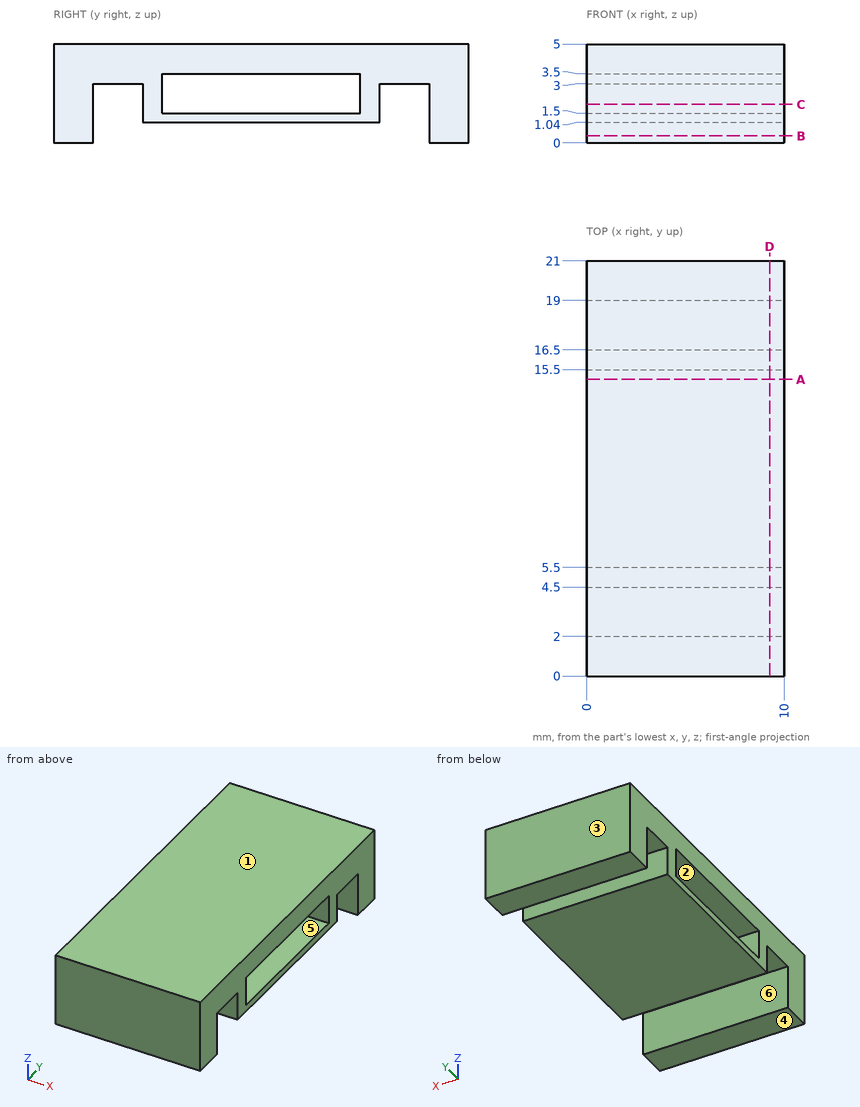
Part print with two shaded views. Sizes in mm from the minimum x, y, z corner. A direction names the side the tool comes from. Round coordinates to 2 decimals unless told otherwise and drop trailing zeros. Order: outer loops, then holes, each group sorted by start corner. A loop starts at its lowest first (then second) coordinate and runs counter-clockwise, first axis right, second up.
(1) Drill centre lines: line 1 (Y direction, x = 8, z = 2.7); line 2 (Y direction, x = 4.25, z = 1.2); line 3 (Z direction, x = 5, y = 10). Where is each one in solid material? Low to high.
(2) Pin check, flat tips, straight feed: pin 1 (0.8 mm diameter, centred on x = 4, y = 3, fed in from -Z); pin 2 (2 mm diameter, centred on x = 3.5, y = 4, fed in from -Z). Stop position of each tip, or through.
(3) Pull direction Z, two halves, no side cores. Call the marked faces 1, 2 and 3: released by +Z, released by -Z, zero draft, split by the parting line, or undercut.
(4) Band-saw the part on B-B (z = 0.35). List the corners of the cut face in (x, y), then the cut area to 3 significant figures.
(5) 3-axis set-ups, long thin cutter, end or side, ignore diameter. For the marked faces 4, 5 and 6: which of +Z, -Z, +X, -X, +Y, -Y reach the whole face in a straight line?
(6) Band-saw the part on D-D (x = 9.25). List the corners of the cut face in (y, z), then the cut area to 3 significant figures.
(7) Band-saw the part on C-C (z = 1.95). List the corners of the cut face in (x, y).
(8) Band-saw the part on A-A (y = 15). List the corners of the cut face in (x, z), then the cut area to 3 significant figures.
Verdict:
1. line 1: y = 0 to 2, 4.5 to 5.5, 15.5 to 16.5, 19 to 21
1. line 2: y = 0 to 2, 4.5 to 16.5, 19 to 21
1. line 3: z = 1.04 to 1.5, 3.5 to 5
2. pin 1: stops at z = 3
2. pin 2: stops at z = 1.04
3. face 1: released by +Z
3. face 2: undercut
3. face 3: zero draft
4. outline: (0, 0) - (10, 0) - (10, 2) - (0, 2) - close; (0, 19) - (10, 19) - (10, 21) - (0, 21) - close
4. area: 40.0 mm2
5. face 4: -Z, +X, -X, +Y, -Y
5. face 5: +X, -X
5. face 6: -Z, +X, -X
6. outline: (0, 0) - (2, 0) - (2, 3) - (4.5, 3) - (4.5, 1.04) - (16.5, 1.04) - (16.5, 3) - (19, 3) - (19, 0) - (21, 0) - (21, 5) - (0, 5) - close; hole (5.5, 1.5) - (15.5, 1.5) - (15.5, 3.5) - (5.5, 3.5) - close
6. area: 57.5 mm2
7. outline: (0, 0) - (10, 0) - (10, 2) - (0, 2) - close; (0, 4.5) - (10, 4.5) - (10, 5.5) - (0, 5.5) - close; (0, 15.5) - (10, 15.5) - (10, 16.5) - (0, 16.5) - close; (0, 19) - (10, 19) - (10, 21) - (0, 21) - close
8. outline: (0, 1.04) - (10, 1.04) - (10, 1.5) - (0, 1.5) - close; (0, 3.5) - (10, 3.5) - (10, 5) - (0, 5) - close
8. area: 19.6 mm2
